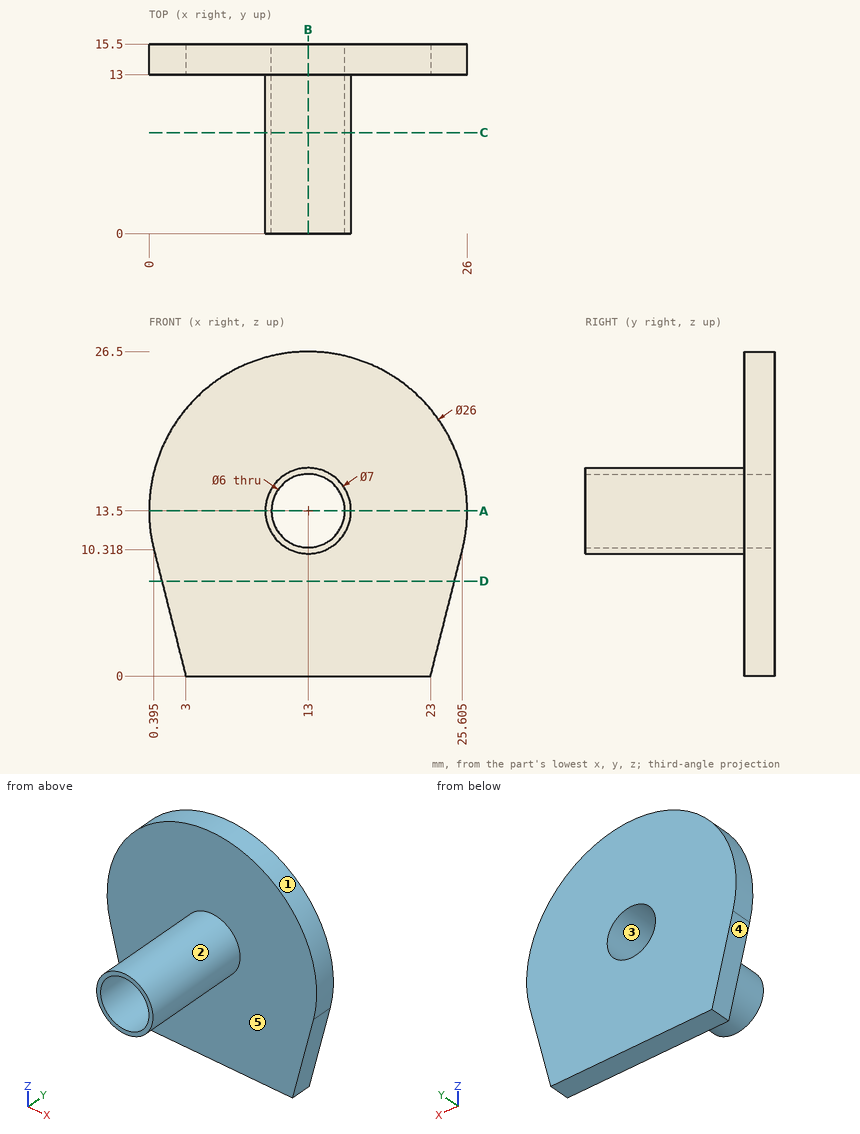
Study the drawing (mm; zero at the part's minimum x, y, z) and answer. A direction names the side the tool comes from. Give positions to 0.01 mm unless a question says otherwise; leave off trailing zeros. Order: outer loops, then holes, each group sorted by start corner. A loop starts at its lowest first (then second) coordinate and runs counter-clockwise, first axis right, second up. Notation, with made-up numbers: (25.25, 8) - (81.25, 8) arc R20 ccw to (81.25, 16) - close; hole circle Ø11 at (25, -28.5). An arc over 180 degrees is marked (long way). Answer in a Markdown table with one row per item. Add a question column.
Q1. The part is cut by section A-A (z = 13.5). Determine the outline of the cut face in (x, y).
Q2. Which of the six approach directions +Z, -Z, +X, -X, +Y, -Y give full straight-line access (tool end or side, diameter ignored) to the marked faces 1 and 2?
Q3. Find the intervals of material crossed by line 1 along Z through (x, y) = (13, 5.25); line 2 along Y through (x, z) = (19.75, 17.5); line 3 along Z through (x, y) = (11.25, 6.5) (1 decimal), in increasing order. Write a range as [from, to].
Q4. For a pull along Z with two mould halves and no side action, classify the marked faces 3, 4 and 5 as released by +Z, released by -Z, zero draft, split by the parting line, or undercut.
Q5. The part is cut by section B-B (x = 13). Determine the outline of the cut face in (y, z).
Q6. The part is cut by section C-C (y = 8.25). Determine the outline of the cut face in (x, z), then the cut area to 3 significant figures.
Q7. Given P1, Ø5.5, axis at x = 13, z = 13.5, coming from the +Y side; P2, Ø8, axis at y = 13, z = 18, coming from the +X side; P3, Ø3, axis at y = 10, z = 17, coming from the -X side; P4, Ø5, axis at y = 12.5, z = 21, coming from the -X side, each flat-ended and moving along its own axis, determine where each tip first touches the part or whether it passes through.
Q8. The part is cut by section D-D (z = 7.75). Determine the outline of the cut face in (x, y).
Determined:
| question | item | result |
|---|---|---|
| 1 | outline | (0, 13) - (9.5, 13) - (9.5, 0) - (10, 0) - (10, 15.5) - (0, 15.5) - close; (16, 0) - (16.5, 0) - (16.5, 13) - (26, 13) - (26, 15.5) - (16, 15.5) - close |
| 2 | face 1 | +Y, -Y |
| 2 | face 2 | -Y |
| 3 | line 1 | z = [10, 10.5], [16.5, 17] |
| 3 | line 2 | y = [13, 15.5] |
| 3 | line 3 | z = [10.5, 11.1], [15.9, 16.5] |
| 4 | face 3 | undercut |
| 4 | face 4 | released by -Z |
| 4 | face 5 | zero draft |
| 5 | outline | (0, 10) - (13, 10) - (13, 0) - (15.5, 0) - (15.5, 10.5) - (0, 10.5) - close; (0, 16.5) - (15.5, 16.5) - (15.5, 26.5) - (13, 26.5) - (13, 17) - (0, 17) - close |
| 6 | outline | circle Ø7 at (13, 13.5); hole circle Ø6 at (13, 13.5) |
| 6 | area | 10.2 mm² |
| 7 | P1 | passes through |
| 7 | P2 | stops at x = 25.99 |
| 7 | P3 | stops at x = 10.13 |
| 7 | P4 | stops at x = 1.02 |
| 8 | outline | (1.04, 13) - (24.96, 13) - (24.96, 15.5) - (1.04, 15.5) - close |
